Input: part model. Units: mm. Frame: model coordinates. Face numbers are marked on the shaded views. A direction names the side the tool comes from. Give positions to 0.01 mm unless a question says otherwise; leave off trailing zeros. Loops run counter-clockwise (first coordinate to the right, second up) from the corner with the lowest first, then second, coordinate; pieces in that order, holes last.
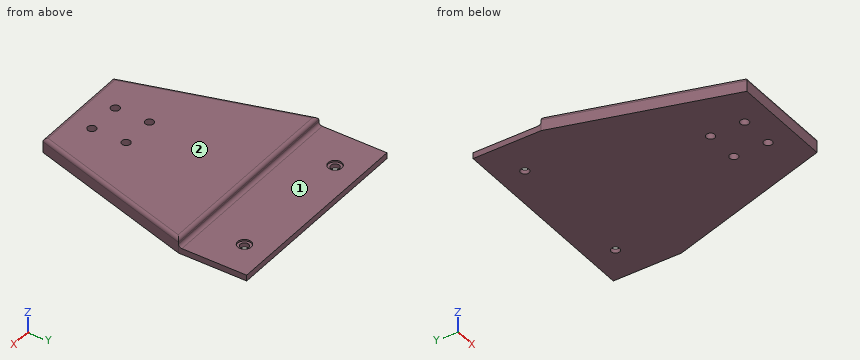
from build123d import *

# Parameters (mm, degrees)
BOSS_EXTRUDE1_DEPTH = 10.795
SKETCH2_W           = 152.4
SKETCH2_H           = 4.445
BOSS_EXTRUDE2_DEPTH = 50.8
SKETCH3_R           = 3.175
CUT_EXTRUDE1_DEPTH  = 495.317625141
FILLET1_R           = 2.54
FILLET2_R           = 2.54
SKETCH4_R           = 5.08
CUT_EXTRUDE2_DEPTH  = 1.27


with BuildPart() as part:
    # Sketch1 → Boss-Extrude1 (new body)
    with BuildSketch(Plane.XY):
        Polygon((228.6, -311.15), (190.5, -438.15), (114.3, -438.15), (76.2, -311.15), align=None)
    extrude(amount=-BOSS_EXTRUDE1_DEPTH)

    # Sketch2 → Boss-Extrude2 (add)
    with BuildSketch(Plane(origin=(0, -311.15, 0), x_dir=(1, 0, 0), z_dir=(0, 1, 0))):
        with Locations((152.4, 8.5725)):
            Rectangle(SKETCH2_W, SKETCH2_H)
    extrude(amount=BOSS_EXTRUDE2_DEPTH)

    # Sketch3 → Cut-Extrude1 (cut, through all)
    with BuildSketch(Plane(origin=(0, 0, -10.795), x_dir=(-1, 0, 0), z_dir=(0, 0, -1))):
        with Locations((-104.775, -279.4)):
            Circle(SKETCH3_R)
        with Locations((-203.2, -279.4)):
            Circle(SKETCH3_R)
        with Locations((-139.7, -393.7)):
            Circle(SKETCH3_R)
        with Locations((-165.1, -393.7)):
            Circle(SKETCH3_R)
        with Locations((-139.7, -419.1)):
            Circle(SKETCH3_R)
        with Locations((-165.1, -419.1)):
            Circle(SKETCH3_R)
    extrude(amount=-CUT_EXTRUDE1_DEPTH, mode=Mode.SUBTRACT)

    # Fillet1
    fillet1_edges = [part.edges().sort_by_distance(p)[0] for p in [
        (152.4, -311.15, -6.35),
    ]]
    fillet(fillet1_edges, radius=FILLET1_R)

    # Fillet2
    fillet2_edges = [part.edges().sort_by_distance(p)[0] for p in [
        (209.55, -374.65, 0),
        (152.4, -438.15, 0),
        (95.25, -374.65, 0),
        (152.4, -311.15, 0),
    ]]
    fillet(fillet2_edges, radius=FILLET2_R)

    # Sketch4 → Cut-Extrude2 (cut)
    with BuildSketch(Plane.XY.offset(-6.35)):
        with Locations((104.775, -279.4)):
            Circle(SKETCH4_R)
        with Locations((203.2, -279.4)):
            Circle(SKETCH4_R)
    extrude(amount=-CUT_EXTRUDE2_DEPTH, mode=Mode.SUBTRACT)


solid = part.part
(1) Ray query, probe 1 along Y at (x, z) = (165.1, -2.25) (3 decimals); probe 2 along X at (y, z) = (-279.4, -8.95) (3 decimals); probe 3 along X at (y, z) = (-279.4, -6.8) (3 decimals). Return the intervals inside material, ascending.
Values follow:
probe 1: y = -438.133 to -422.275, -415.925 to -396.875, -390.525 to -311.167
probe 2: x = 76.2 to 101.6, 107.95 to 200.025, 206.375 to 228.6
probe 3: x = 76.2 to 99.695, 109.855 to 198.12, 208.28 to 228.6
(2) Pin query (flat end, axial travel): pin 1 Ø7.5 at (x, y) = (203.2, -279.4) entering from -Z (3 decimals); pin 2 Ø5 at (x, y) = (104.775, -279.4) entering from -Z; pin 3 Ø13 at (x, y) = (203.2, -279.4) entering from +Z; pin 4 Ø3 at (y, z) = (-363, -4.5) entering from +X (3 decimals). Return the tip coordinate at first contact, or that it passes through.
Values follow:
pin 1: stops at z = -10.795
pin 2: passes through
pin 3: stops at z = -6.35
pin 4: stops at x = 213.495
(3) Cut plane B-B (y = -393.7). Count the separate pieces of the cut face and the enclosed holes in it, and give its area (3 significant figures).
Values follow:
separate pieces: 3
enclosed holes: 0
area: 970 mm2
(4) Cut plane A-A (x = 139.7). Return the cut outline in (y, z) (3 decimals), and give its area (3 significant figures).
Values follow:
outline: (-438.15, -10.795) - (-422.275, -10.795) - (-422.275, 0) - (-435.61, 0) arc R2.54 ccw to (-438.15, -2.54) - close; (-415.925, -10.795) - (-396.875, -10.795) - (-396.875, 0) - (-415.925, 0) - close; (-390.525, -10.795) - (-260.35, -10.795) - (-260.35, -6.35) - (-308.61, -6.35) arc R2.54 cw to (-311.15, -3.81) - (-311.15, -2.54) arc R2.54 ccw to (-313.69, 0) - (-390.525, 0) - close
area: 1,460 mm2
(5) Reachability of the marked faces 1 and 2 from +Z, -Z, +X, -X, +Y, -Y: full face, straight path, thin tool, end or side. Return the list, or none.
Values follow:
face 1: +Z, +X, -X, +Y
face 2: +Z, +X, -X, +Y, -Y
